Could you check a few things on this model? Use its own coordinates, in mm. Face numbers are marked on the shaded views. A direction names the side the tool comes from. Round coordinates to 2 decimals unless told otherwise and drop trailing zeros. Order: outer loops, then holes, each group sorted by start corner. A loop starts at its lowest first (then second) coordinate and runs counter-clockwise, first axis right, second up. Notation, with made-up numbers: (6.25, 52.25) - (22.25, 52.25) arc R5 ccw to (22.25, 56.25) - close; hole circle Ø11 at (-32.75, 84.5). An arc over 180 degrees is marked (long way). Use one line per item in the form item = value.
from build123d import *

# Parameters (mm, degrees)
SKETCH_3_R          = 5.1
EXTRUDE_1_DEPTH     = 4.8
SKETCH_4_W          = 11
SKETCH_4_H          = 15.8
EXTRUDE_2_DEPTH     = 1
SKETCH_5_R          = 1.5
EXTRUDE_3_DEPTH     = 10.8
CUT_EXTRUDE_1_DEPTH = 10.8
FILLET_1_R          = 0.6
SKETCH_8_R          = 3
CUT_EXTRUDE_2_DEPTH = 4.8
SKETCH_9_R          = 1
CUT_EXTRUDE_3_DEPTH = 1
SKETCH_10_W         = 3
SKETCH_10_H         = 15.8
EXTRUDE_4_DEPTH     = 7
CHAMFER_1_SIZE      = 3
SKETCH_11_W         = 2.584868303
SKETCH_11_H         = 3
EXTRUDE_5_DEPTH     = 10
CHAMFER_4_SIZE      = 1.6584
CHAMFER_5_SIZE      = 2
CHAMFER_6_SIZE      = 2
EXTRUDE_6_DEPTH     = 2.7


# Read off the part's stored shape, not the designer's step: Бобышка-Вытянуть6
with BuildPart() as part:
    # Эскиз3 → Бобышка-Вытянуть1 (new body)
    with BuildSketch(Plane.XY):
        with Locations((0, -6.52)):
            Circle(SKETCH_3_R)
    extrude(amount=EXTRUDE_1_DEPTH)

    # Эскиз4 → Бобышка-Вытянуть2 (add)
    with BuildSketch(Plane(origin=(0, 0, 0), x_dir=(-1, 0, 0), z_dir=(0, 0, -1))):
        with Locations((0, -7.22)):
            Rectangle(SKETCH_4_W, SKETCH_4_H)
    extrude(amount=EXTRUDE_2_DEPTH)

    # Эскиз5 → Бобышка-Вытянуть3 (add)
    with BuildSketch(Plane(origin=(0, 0, -1), x_dir=(-1, 0, 0), z_dir=(0, 0, -1))):
        with Locations(Location((-4.415131697, -8.961534596, 0), (0, 0, 136.323092078))):
            Circle(SKETCH_5_R)
    extrude(amount=EXTRUDE_3_DEPTH)

    # Эскиз6 → Вырез-Вытянуть1 (cut)
    with BuildSketch(Plane.XY.offset(-1)):
        with BuildLine():
            Line((5.5, -7.925648132), (5.5, -9.997421059))
            ThreePointArc((5.5, -9.997421059), (5.915131697, -8.961534596), (5.5, -7.925648132))
        make_face()
    extrude(amount=-CUT_EXTRUDE_1_DEPTH, mode=Mode.SUBTRACT)

    # Скругление1
    fillet_1_edges = [part.edges().sort_by_distance(p)[0] for p in [
        (-5.1, -6.52, 4.8),
    ]]
    fillet(fillet_1_edges, radius=FILLET_1_R)

    # Эскиз8 → Вырез-Вытянуть2 (cut)
    with BuildSketch(Plane.XY.offset(4.8)):
        with Locations((0, -6.52)):
            Circle(SKETCH_8_R)
    extrude(amount=-CUT_EXTRUDE_2_DEPTH, mode=Mode.SUBTRACT)

    # Эскиз9 → Вырез-Вытянуть3 (cut)
    with BuildSketch(Plane.XY):
        with Locations((0, -6.52)):
            Circle(SKETCH_9_R)
    extrude(amount=-CUT_EXTRUDE_3_DEPTH, mode=Mode.SUBTRACT)

    # Эскиз10 → Бобышка-Вытянуть4 (add)
    with BuildSketch(Plane(origin=(0, 0, -1), x_dir=(-1, 0, 0), z_dir=(0, 0, -1))):
        with Locations((-4, -7.22)):
            Rectangle(SKETCH_10_W, SKETCH_10_H)
    extrude(amount=EXTRUDE_4_DEPTH)

    # Фаска1
    chamfer_1_edges = [part.edges().sort_by_distance(p)[0] for p in [
        (4, -15.12, -8),
        (4, 0.68, -8),
    ]]
    chamfer(chamfer_1_edges, length=CHAMFER_1_SIZE)

    # Эскиз11 → Бобышка-Вытянуть5 (add)
    with BuildSketch(Plane(origin=(0, 0, -11.8), x_dir=(-1, 0, 0), z_dir=(0, 0, -1))):
        with Locations((-4.207565848, -8.961534596)):
            Rectangle(SKETCH_11_W, SKETCH_11_H)
    extrude(amount=-EXTRUDE_5_DEPTH)

    # Фаска4
    chamfer_4_edges = [part.edges().sort_by_distance(p)[0] for p in [
        (4.207565848, -10.461534596, -8),
    ]]
    chamfer(chamfer_4_edges, length=CHAMFER_4_SIZE)

    # Фаска5
    chamfer_5_edges = [part.edges().sort_by_distance(p)[0] for p in [
        (4.207565848, -7.461534596, -8),
    ]]
    chamfer(chamfer_5_edges, length=CHAMFER_5_SIZE)

    # Фаска6
    # the kernel refuses this chamfer: 2 mm, written as the material it adds along each edge
    with BuildSketch(Plane(origin=(2.915131697, -0.31816862, -8), x_dir=(-0.9996219169112968, 0, 0.027495876610586487), z_dir=(0, -1, 0))) as chamfer_6_piece_1_section:
        Polygon((CHAMFER_6_SIZE * 0.999621916911, CHAMFER_6_SIZE * 0.0274958766106), (-CHAMFER_6_SIZE * 0.0274958766106, CHAMFER_6_SIZE * 0.999621916911), (0, 0), align=None)
    chamfer_6_piece_1 = extrude(amount=16.945131952, mode=Mode.PRIVATE)
    chamfer_6_piece_1 = split(chamfer_6_piece_1, bisect_by=Plane(origin=(2.709078012, -6.449232398, -8.987697802), z_dir=(0, -0.7071067811865476, 0.7071067811865476)), keep=Keep.TOP, mode=Mode.PRIVATE)
    chamfer_6_piece_1 = split(chamfer_6_piece_1, bisect_by=Plane(origin=(2.709078012, -10.461534596, -8.650263736), z_dir=(0, 1, 0)), keep=Keep.TOP, mode=Mode.PRIVATE)
    chamfer_6_piece_1 = split(chamfer_6_piece_1, bisect_by=Plane(origin=(2.5, -6.786666464, -8.650263736), z_dir=(1, 0, 0)), keep=Keep.TOP, mode=Mode.PRIVATE)
    add(chamfer_6_piece_1)
    with BuildSketch(Plane(origin=(2.915131697, -0.31816862, -8), x_dir=(-0.9996219169112968, 0, 0.027495876610586487), z_dir=(0, -1, 0))) as chamfer_6_piece_2_section:
        Polygon((CHAMFER_6_SIZE * 0.999621916911, CHAMFER_6_SIZE * 0.0274958766106), (-CHAMFER_6_SIZE * 0.0274958766106, CHAMFER_6_SIZE * 0.999621916911), (0, 0), align=None)
    chamfer_6_piece_2 = extrude(amount=16.945131952, mode=Mode.PRIVATE)
    chamfer_6_piece_2 = split(chamfer_6_piece_2, bisect_by=Plane(origin=(2.70758781, -10.461534596, -8.552675921), z_dir=(0, -1, 0)), keep=Keep.TOP, mode=Mode.PRIVATE)
    chamfer_6_piece_2 = split(chamfer_6_piece_2, bisect_by=Plane(origin=(2.70758781, -11.290827655, -8.829106941), z_dir=(0, 0.7071067811865476, 0.7071067811865476)), keep=Keep.TOP, mode=Mode.PRIVATE)
    chamfer_6_piece_2 = split(chamfer_6_piece_2, bisect_by=Plane(origin=(2.5, -11.014396635, -8.552675921), z_dir=(1, 0, 0)), keep=Keep.TOP, mode=Mode.PRIVATE)
    add(chamfer_6_piece_2)

    # Бобышка-Вытянуть6 outline → Бобышка-Вытянуть6 (add)
    with BuildSketch(Plane(origin=(5.5, 0, 0), x_dir=(0, 0, -1), z_dir=(1, 0, 0))):
        Polygon((10, -7.461534596), (8, -5.461534596), (8, -2.32), (5, 0.68), (0, 0.68), (0, -15.12), (5, -15.12), (8, -12.12), (9.6584, -10.461534596), (10, -10.461534596), align=None)
    extrude(amount=EXTRUDE_6_DEPTH)


solid = part.part
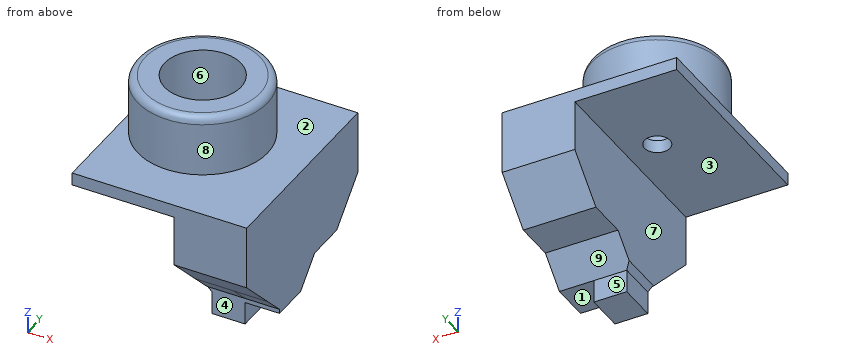
Item 1: For the marked faces 1, 2, 3, 4 and 5, which set-ups out of +Z, -Z, +X, -X, +Y, -Y let a thin tool reach every point of the face, with its end or its side?
Found:
face_1 = -Z, +X, +Y, -Y
face_2 = +Z
face_3 = -Z, -X, +Y, -Y
face_4 = -Z, +X, -X, -Y
face_5 = -Z, +X, -X, +Y
Item 2: Imagine slicing it at A-A on x = 0. Please give me the cut outline in (y, z), plus the area to 3 significant figures.
Found:
outline = (-15.12, -1) - (-7.52, -1) - (-7.52, 0) - (-9.52, 0) - (-9.52, 4.8) - (-11.02, 4.8) arc R0.6 ccw to (-11.62, 4.2) - (-11.62, 0) - (-15.12, 0) - close; (-5.52, -1) - (0.68, -1) - (0.68, 0) - (-1.42, 0) - (-1.42, 4.2) arc R0.6 ccw to (-2.02, 4.8) - (-3.52, 4.8) - (-3.52, 0) - (-5.52, 0) - close
area = 33.8 mm2
Item 3: If we mould it in two halves opening along X, with no side actions, what happens to the marked faces 6, 7, 8 and 9? For each: released by +X, released by -X, zero draft, split by the parting line, or undercut.
Found:
face_6 = undercut
face_7 = released by -X
face_8 = split by the parting line
face_9 = zero draft
Item 4: I need wall thicknesses on L1, parallel to Y at x = 0, z = 2.3; L2, parallel to Y at x = 0, z = -0.4; L3, parallel to Z at x = 7.25, y = -7.5. Which ranges of each line are inside material? Lowest first, please.
Found:
L1 = -11.62 to -9.52, -3.52 to -1.42
L2 = -15.12 to -7.52, -5.52 to 0.68
L3 = -10 to 0
Item 5: Will these pins go through, and if not, where does the flat tip stop? P1, Ø0.9, axis at y = -9, z = -11, coming from the -X side; P2, Ø2.5, axis at x = 6.5, y = -3, coming from the -Z side; P3, Ø1.1, axis at x = 4, z = -11, coming from the -Y side.
Found:
P1 = 2.92
P2 = -8
P3 = -10.46
Item 6: Imagine slicing it at C-C on y = -6.52. Please give me the cut outline in (x, z), plus the area to 3 significant figures.
Found:
outline = (-5.5, -1) - (-1, -1) - (-1, 0) - (-3, 0) - (-3, 4.8) - (-4.5, 4.8) arc R0.6 ccw to (-5.1, 4.2) - (-5.1, 0) - (-5.5, 0) - close; (1, -1) - (2.5, -1) - (2.5, -9.06) - (8.2, -9.06) - (8.2, 0) - (5.1, 0) - (5.1, 4.2) arc R0.6 ccw to (4.5, 4.8) - (3, 4.8) - (3, 0) - (1, 0) - close
area = 77.6 mm2
Item 7: Imagine slicing it at D-D on z = -1.25. Please give me the cut outline in (x, y).
Found:
outline = (2.5, -15.12) - (8.2, -15.12) - (8.2, 0.68) - (2.5, 0.68) - close
Item 8: Imagine slicing it at B-B on y = -14. Please give me the cut outline in (x, z), plus the area to 3 significant figures.
Found:
outline = (-5.5, -1) - (2.5, -1) - (2.5, -6.12) - (8.2, -6.12) - (8.2, 0) - (-5.5, 0) - close
area = 42.9 mm2
